```python
from build123d import *

# Parameters (mm, degrees)
F0_W     = 14
F0_H     = 14
F1_DEPTH = 3


# Not quite as in the source:
# - a feature names something its author has since deleted; it is built from what else it names


with BuildPart() as f1:
    # F0 (on Top) → F1 (new body)
    with BuildSketch(Plane.XY):
        with BuildLine():
            Line((2.625, -8), (8, -8))
            Line((8, -8), (8, 8))
            Line((8, 8), (2.625, 8))
            Line((2.625, 8), (2, 8))
            Line((2, 8), (1.7001838136, 8))
            ThreePointArc((1.7001838136, 8), (0, 7.375), (-1.7001838136, 8))
            Line((-1.7001838136, 8), (-2, 8))
            Line((-2, 8), (-2.625, 8))
            Line((-2.625, 8), (-8, 8))
            Line((-8, 8), (-8, -8))
            Line((-8, -8), (-2.625, -8))
            Line((-2.625, -8), (-2, -8))
            Line((-2, -8), (-1.7001838136, -8))
            ThreePointArc((-1.7001838136, -8), (0, -7.375), (1.7001838136, -8))
            Line((1.7001838136, -8), (2, -8))
            Line((2, -8), (2.625, -8))
        make_face()
        Rectangle(F0_W, F0_H, mode=Mode.SUBTRACT)
        with BuildLine():
            Line((2.625, -10), (2.625, -8))
            Line((2.625, -8), (2, -8))
            Line((2, -8), (2, -8.2998161864))
            ThreePointArc((2, -8.2998161864), (2.4638004181, -9.0942889534), (2.625, -10))
        make_face()
        with BuildLine():
            Line((2, -8.2998161864), (2, -8))
            Line((2, -8), (1.7001838136, -8))
            ThreePointArc((1.7001838136, -8), (1.8561553006, -8.1438446994), (2, -8.2998161864))
        make_face()
        with BuildLine():
            ThreePointArc((2, -11.7001838136), (2.4638004181, -10.9057110466), (2.625, -10))
            ThreePointArc((2.625, -10), (2.4638004181, -9.0942889534), (2, -8.2998161864))
            Line((2, -8.2998161864), (2, -11.7001838136))
        make_face()
        with BuildLine():
            Line((2, 8), (2.625, 8))
            Line((2.625, 8), (2.625, 10))
            ThreePointArc((2.625, 10), (2.382604406, 8.8982644398), (1.7001838136, 8))
            Line((1.7001838136, 8), (2, 8))
        make_face()
        with BuildLine():
            ThreePointArc((2, -8.2998161864), (1.8561553006, -8.1438446994), (1.7001838136, -8))
            Line((1.7001838136, -8), (0, -8))
            Line((0, -8), (-1.7001838136, -8))
            ThreePointArc((-1.7001838136, -8), (-2.382604406, -8.8982644398), (-2.625, -10))
            ThreePointArc((-2.625, -10), (-0.9057110466, -12.4638004181), (2, -11.7001838136))
            Line((2, -11.7001838136), (2, -8.2998161864))
        make_face()
        with BuildLine():
            ThreePointArc((1.5, -10), (-1.0606601718, -11.0606601718), (0, -8.5))
            ThreePointArc((0, -8.5), (1.0606601718, -8.9393398282), (1.5, -10))
        make_face(mode=Mode.SUBTRACT)
        with BuildLine():
            Line((0, -8), (1.7001838136, -8))
            ThreePointArc((1.7001838136, -8), (0, -7.375), (-1.7001838136, -8))
            Line((-1.7001838136, -8), (0, -8))
        make_face()
        with BuildLine():
            ThreePointArc((1.7001838136, 8), (2.382604406, 8.8982644398), (2.625, 10))
            ThreePointArc((2.625, 10), (0, 12.625), (-2.625, 10))
            ThreePointArc((-2.625, 10), (-2.382604406, 8.8982644398), (-1.7001838136, 8))
            Line((-1.7001838136, 8), (0, 8))
            Line((0, 8), (1.7001838136, 8))
        make_face()
        with BuildLine():
            ThreePointArc((1.5, 10), (1.0606601718, 8.9393398282), (0, 8.5))
            ThreePointArc((0, 8.5), (-1.0606601718, 11.0606601718), (1.5, 10))
        make_face(mode=Mode.SUBTRACT)
        with BuildLine():
            ThreePointArc((-2.625, -10), (-2.382604406, -8.8982644398), (-1.7001838136, -8))
            Line((-1.7001838136, -8), (-2, -8))
            Line((-2, -8), (-2.625, -8))
            Line((-2.625, -8), (-2.625, -10))
        make_face()
        with BuildLine():
            ThreePointArc((-1.7001838136, 8), (0, 7.375), (1.7001838136, 8))
            Line((1.7001838136, 8), (0, 8))
            Line((0, 8), (-1.7001838136, 8))
        make_face()
        with BuildLine():
            ThreePointArc((-1.7001838136, 8), (-2.382604406, 8.8982644398), (-2.625, 10))
            Line((-2.625, 10), (-2.625, 8))
            Line((-2.625, 8), (-2, 8))
            Line((-2, 8), (-1.7001838136, 8))
        make_face()
    extrude(amount=F1_DEPTH)


solid = f1.part
```
Here's how the part is built. I have some questions about the finished solid (model axes, mm). A direction names the side the tool comes from. Coordinates: 2 decimals unless noted, no trailing zeros. Order: outer loops, then holes, each group sorted by start corner. A loop starts at its lowest first (then second) coordinate and runs counter-clockwise, first axis right, second up. Notation, with made-up numbers: (69.5, 65) - (99.5, 65) arc R17 cw to (99.5, 78) - close; hole circle Ø2 at (48, 8). An arc over 180 degrees is marked (long way). One line per question, with ' | ' between items. Start each with the question number.
1. Which directions (+Z, -Z, +X, -X, +Y, -Y) give clear straight access to the entire face, cutting with the end or side of a thin tool? Please do faces 5 (the flat face through (-2.625, 9, 1)), 6 (the flat face through (2.625, -9, 1)), 7 (the flat face through (0, 7, 1)), 8 (the flat face through (-2.625, -9, 1)).
2. If we mould it in two halves opening along X, with no side actions, what happens to faces 1 (the flat face through (-5, 8, 1)), 2 (the flat face through (7, 0, 1)), 3 (the flat face through (0, -7, 1)), 4 (the flat face through (2.625, 9, 1))? For each: released by +X, released by -X, zero draft, split by the parting line, or undercut.
3. If we section it at C-C (x = 0.5): Write out the boundary of the cut face in (y, z), and give its area (3 significant figures).
4. If we section it at B-B (y = -1.75): Write out the boundary of the cut face in (x, z), and give its area (3 significant figures).
5. Please list where these lines run through material, in increasing order: line 1 along X through (y, z) = (2.5, 2.15); line 2 along X through (y, z) = (-10, 1.1) (3 decimals). Write a range as [from, to].
6. I'm going to push flat-ended pins straight in: pin 1 Ø1 at (y, z) = (9.5, 2) entering from -X (3 decimals); pin 2 Ø1.5 at (x, z) = (2.5, 2) entering from +Y; pin 3 Ø6 at (x, y) = (3, 2) entering from +Z; pin 4 Ø1.5 at (x, z) = (5.5, 1) entering from +Y. Where does each tip first touch, or does it pass through?
7. If we section it at A-A (z = 0.25): Write out the boundary of the cut face in (x, y) (3 decimals), and give its area (3 significant figures).
8. If we section it at D-D (y = 11.25): Write out the boundary of the cut face in (x, z).
Model answer:
1) face 5: +Z, -Z, -X, +Y | face 6: +Z, -Z, +X, -Y | face 7: +Z, -Z | face 8: +Z, -Z, -X, -Y
2) face 1: zero draft | face 2: undercut | face 3: undercut | face 4: released by +X
3) outline: (-12.58, 0) - (-11.41, 0) - (-11.41, 3) - (-12.58, 3) - close; (-8.59, 0) - (-7, 0) - (-7, 3) - (-8.59, 3) - close; (7, 0) - (8.59, 0) - (8.59, 3) - (7, 3) - close; (11.41, 0) - (12.58, 0) - (12.58, 3) - (11.41, 3) - close | area: 16.5 mm²
4) outline: (-8, 0) - (-7, 0) - (-7, 3) - (-8, 3) - close; (7, 0) - (8, 0) - (8, 3) - (7, 3) - close | area: 6.00 mm²
5) line 1: x = [-8, -7], [7, 8] | line 2: x = [-2.625, -1.5], [1.5, 2.625]
6) pin 1: stops at x = -2.625 | pin 2: stops at y = 11.96 | pin 3: passes through | pin 4: stops at y = 8
7) outline: (-8, -8) - (-2.625, -8) - (-2.625, -10) arc R2.625 ccw to (2.625, -10) - (2.625, -8) - (8, -8) - (8, 8) - (2.625, 8) - (2.625, 10) arc R2.625 ccw to (-2.625, 10) - (-2.625, 8) - (-8, 8) - close; hole (-7, -7) - (7, -7) - (7, 7) - (-7, 7) - close; hole circle Ø3 at (0, -10); hole circle Ø3 at (0, 10) | area: 88.5 mm²
8) outline: (-2.31, 0) - (-0.83, 0) - (-0.83, 3) - (-2.31, 3) - close; (0.83, 0) - (2.31, 0) - (2.31, 3) - (0.83, 3) - close
